Build history of the part. All positions in model axes, mm. Face numbers are marked on the shaded views. Coordinates: 2 decimals unless noted, no trailing zeros. Write each loop counter-clockwise with the first axis right and the second up, starting at its lowest first coordinate (ties: lowest second). Pieces come first, ordered by that corner, then holes.
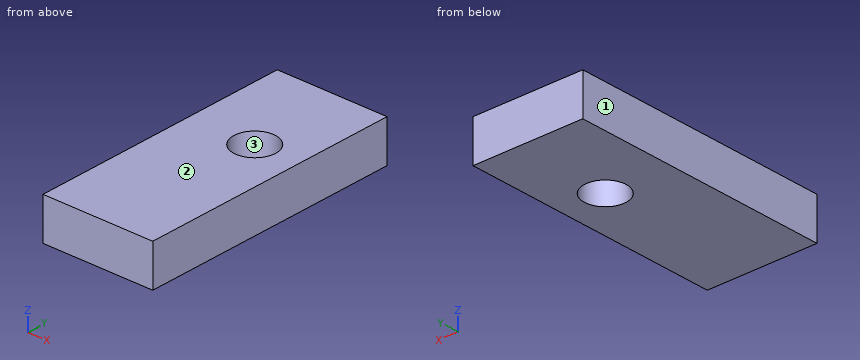
Autodesk Inventor part; units mm, degrees
ref_plane "YZ Plane" through (0, 0, 0) normal (1, 0, 0) x (0, 1, 0)
ref_plane "XZ Plane" through (0, 0, 0) normal (0, 1, 0) x (-1, 0, 0)
ref_plane "XY Plane" through (0, 0, 0) normal (0, 0, 1) x (1, 0, 0)
sketch "Sketch1" plane through (0, 0, 0) normal (0, 0, 1) x (1, 0, 0)
  line L0 (0, 20) -> (0, 0)
  circle A0 centre (5, 12.5) radius 1.6
  line L1 (8.4, 20) -> (8.4, 0)
  line L2 (0, 20) -> (8.4, 20)
  line L3 (0, 0) -> (8.4, 0)
  dimension "d2" = 3.2
  dimension "d3" = 5
  dimension "d12" = 8.4
  dimension "d14" = 7.5
  dimension "d15" = 8.4
  dimension "d16" = 20
extrude "Extrusion1" add sketch "Sketch1" along normal blind 3.175
equation "\"d12\" = d13"
properties part number "Effector_ZProbe_B"
1. Saw through at C-C on z = 1.6. List the corners of the cut face in (x, y).
Computed values:
outline: (0, 0) - (8.4, 0) - (8.4, 20) - (0, 20) - close; hole circle Ø3.2 at (5, 12.5)
2. Probe line 1 along Y through (x, z) = (5, 0.5); line 2 along X through (y, z) = (12.75, 2.4); line 3 along Y through (x, z) = (6.25, 0.55). List the from-to ranges inside material, lowest first.
Computed values:
line 1: y = 0 to 10.9, 14.1 to 20
line 2: x = 0 to 3.42, 6.58 to 8.4
line 3: y = 0 to 11.5, 13.5 to 20
3. Saw through at A-A on y = 12.5. List the corners of the cut face in (x, z) (3 decimals).
Computed values:
outline: (0, 0) - (3.4, 0) - (3.4, 3.175) - (0, 3.175) - close; (6.6, 0) - (8.4, 0) - (8.4, 3.175) - (6.6, 3.175) - close
4. Saw through at B-B on x = 5. List the corners of the cut face in (y, z) (3 decimals), plus the area to 3 significant figures.
Computed values:
outline: (0, 0) - (10.9, 0) - (10.9, 3.175) - (0, 3.175) - close; (14.1, 0) - (20, 0) - (20, 3.175) - (14.1, 3.175) - close
area: 53.3 mm2
5. Mould opens along X. For the marked faces 1, 2 and 3 say: +X half, -X half, draft (parallel to the pull), parting line (faces both ways), or undercut.
Computed values:
face 1: -X half
face 2: draft
face 3: undercut
